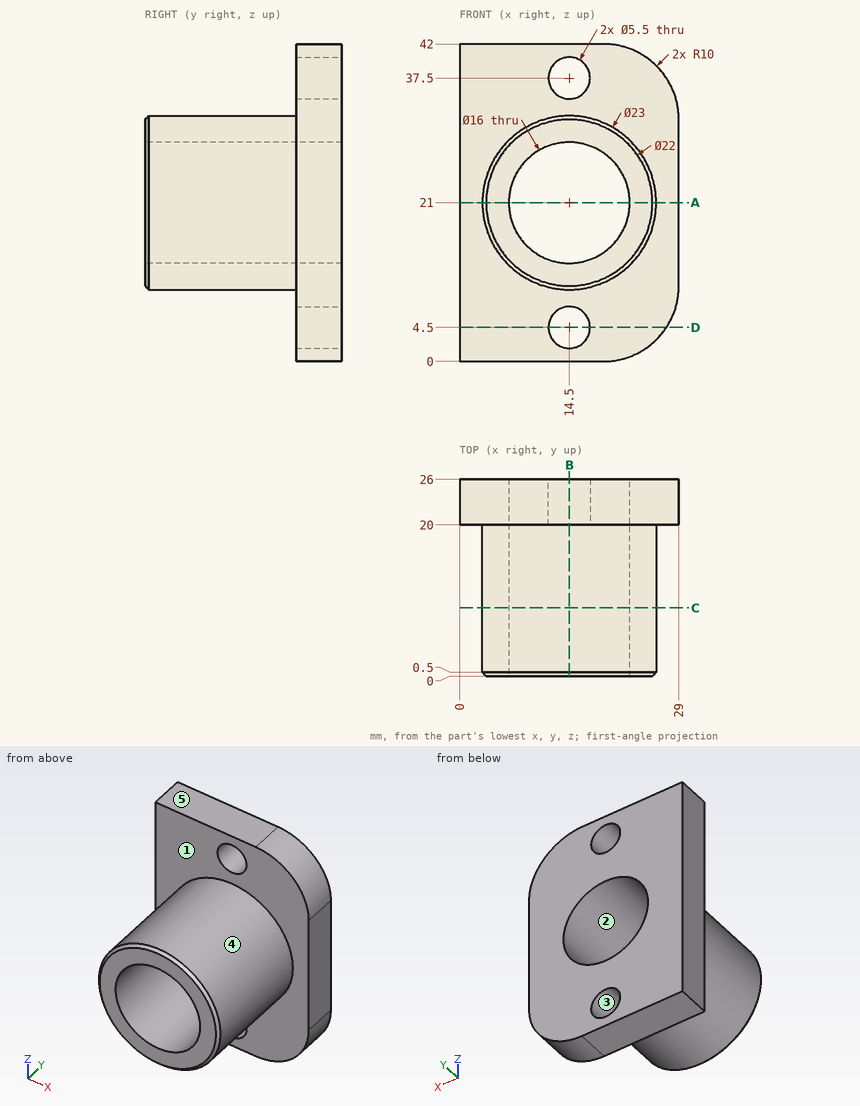
Print and shaded views of the part. All mm, measured from the part's lowest x, y and z. A direction names the side the tool comes from. Round coordinates to 2 decimals unless told otherwise and drop trailing zeros. Order: outer loops, then holes, each group sorted by start corner. A loop starts at its lowest first (then second) coordinate and runs counter-clockwise, first axis right, second up. Notation, with made-up numbers: (-23, -6) - (34, -6) arc R21 ccw to (34, 8) - close; hole circle Ø9 at (18.25, -34). An arc over 180 degrees is marked (long way). Use a Markdown table: item, result.
1) Saw through at A-A on z = 21. Write the cut outline in (x, y).
Recorded:
| item | result |
|---|---|
| outline | (0, 20) - (3, 20) - (3, 0.5) - (3.5, 0) - (6.5, 0) - (6.5, 26) - (0, 26) - close; (22.5, 0) - (25.5, 0) - (26, 0.5) - (26, 20) - (29, 20) - (29, 26) - (22.5, 26) - close |
2) Tool access for the marked faces 1 and 2: list every direction of +Z, -Z, +X, -X, +Y, -Y with a clear straight run to the whole face (end or side of a thin tool).
Recorded:
| item | result |
|---|---|
| face 1 | -Y |
| face 2 | +Y, -Y |
3) Saw through at C-C on y = 9. Write the cut outline in (x, z), and give its area (3 significant figures).
Recorded:
| item | result |
|---|---|
| outline | circle Ø23 at (14.5, 21); hole circle Ø16 at (14.5, 21) |
| area | 214 mm² |
4) Flat gauge pins, fed straight in: pin 1 Ø8 at (y, z) = (5, 22) entering from +X; pin 2 Ø5 at (x, z) = (14.5, 37.5) entering from +Y; pin 3 Ø3 at (y, z) = (8.5, 16) entering from -X; pin 4 Ø6 at (x, z) = (8.5, 35) entering from -Y. Where does each tip first touch, or does it go through?
Recorded:
| item | result |
|---|---|
| pin 1 | stops at x = 26 |
| pin 2 | passes through |
| pin 3 | stops at x = 3.55 |
| pin 4 | stops at y = 20 |
5) Saw through at D-D on z = 4.5. Write the cut outline in (x, y).
Recorded:
| item | result |
|---|---|
| outline | (0, 20) - (11.75, 20) - (11.75, 26) - (0, 26) - close; (17.25, 20) - (27.35, 20) - (27.35, 26) - (17.25, 26) - close |
6) Saw through at B-B on x = 14.5. Write the cut outline in (y, z), and give its area (3 significant figures).
Recorded:
| item | result |
|---|---|
| outline | (0, 10) - (0.5, 9.5) - (20, 9.5) - (20, 7.25) - (26, 7.25) - (26, 13) - (0, 13) - close; (0, 29) - (26, 29) - (26, 34.75) - (20, 34.75) - (20, 32.5) - (0.5, 32.5) - (0, 32) - close; (20, 0) - (26, 0) - (26, 1.75) - (20, 1.75) - close; (20, 40.25) - (26, 40.25) - (26, 42) - (20, 42) - close |
| area | 230 mm² |
7) Pull direction X, two halves, no side cores. Call the marked faces 3, 4 and 5: pulls with the +X half, pulls with the -X half, needs draft (parallel to the pull), parting line crosses it, or undercut.
Recorded:
| item | result |
|---|---|
| face 3 | undercut |
| face 4 | parting line crosses it |
| face 5 | needs draft |
8) Wall check: L1, parallel to Z at x = 14.5, y = 21.4; L2, parallel to Z at x = 14.5, y = 11.75; L3, parallel to Y at x = 17.25, z = 8. Give the ranges that are in metal, low to high.
Recorded:
| item | result |
|---|---|
| L1 | z = 0 to 1.75, 7.25 to 13, 29 to 34.75, 40.25 to 42 |
| L2 | z = 9.5 to 13, 29 to 32.5 |
| L3 | y = 20 to 26 |
